from build123d import *

# Parameters (mm, degrees)
SKETCH_1_W          = 60
SKETCH_1_H          = 110
EXTRUDE_1_DEPTH     = 10
SKETCH_2_W          = 10
SKETCH_2_H          = 110
EXTRUDE_2_DEPTH     = 85
CUT_EXTRUDE_1_DEPTH = 85
SKETCH_4_R          = 26
EXTRUDE_3_DEPTH     = 21
CUT_EXTRUDE_2_DEPTH = 42
SKETCH_6_R          = 32
EXTRUDE_4_DEPTH     = 10
SKETCH_7_R          = 17.5
CUT_EXTRUDE_3_DEPTH = 81


with BuildPart() as part:
    # 스케치1 → 보스-돌출1 (new body)
    with BuildSketch(Plane(origin=(0, 0, 0), x_dir=(1, 0, 0), z_dir=(0, 1, 0))):
        Rectangle(SKETCH_1_W, SKETCH_1_H)
    extrude(amount=EXTRUDE_1_DEPTH)

    # 스케치2 → 보스-돌출2 (add)
    with BuildSketch(Plane(origin=(0, 10, 0), x_dir=(1, 0, 0), z_dir=(0, 1, 0))):
        Rectangle(SKETCH_2_W, SKETCH_2_H)
    extrude(amount=EXTRUDE_2_DEPTH)

    # 스케치3 → 컷-돌출1 (cut)
    with BuildSketch(Plane(origin=(5, 0, 0), x_dir=(0, 0, -1), z_dir=(1, 0, 0))):
        Polygon((-55, 10), (-1.927245104, 101.924707978), (-74.670847317, 101.924707978), (-74.670847317, 10), align=None)
    cut_extrude_1 = extrude(amount=-CUT_EXTRUDE_1_DEPTH, mode=Mode.SUBTRACT)

    # 대칭 복사1: 컷-돌출1 across plane
    add(cut_extrude_1.mirror(Plane.XY), mode=Mode.SUBTRACT)

    # 스케치4 → 보스-돌출3 (add, symmetric)
    with BuildSketch(Plane(origin=(0, 0, 0), x_dir=(0, 0, -1), z_dir=(1, 0, 0))):
        with Locations((0, 66)):
            Circle(SKETCH_4_R)
    extrude(amount=EXTRUDE_3_DEPTH, both=True)

    # 스케치5 → 컷-돌출2 (cut)
    with BuildSketch(Plane(origin=(21, 0, 0), x_dir=(0, 0, -1), z_dir=(1, 0, 0))):
        with BuildLine():
            Line((-16.854508663, 85.797109328), (-12.442891348, 105.747158049))
            Line((-12.442891348, 105.747158049), (16.049526521, 102.320854634))
            Line((16.049526521, 102.320854634), (20.027337967, 82.58028148))
            ThreePointArc((20.027337967, 82.58028148), (2.259138508, 91.901665838), (-16.854508663, 85.797109328))
        make_face()
    extrude(amount=-CUT_EXTRUDE_2_DEPTH, mode=Mode.SUBTRACT)

    # 스케치6 → 보스-돌출4 (add)
    with BuildSketch(Plane(origin=(21, 0, 0), x_dir=(0, 0, -1), z_dir=(1, 0, 0))):
        with Locations((0, 66)):
            Circle(SKETCH_6_R)
    extrude_4 = extrude(amount=EXTRUDE_4_DEPTH)

    # 대칭 복사2: 보스-돌출4 across plane
    add(extrude_4.mirror(Plane(origin=(0, 0, 0), x_dir=(0, 0, 1), z_dir=(1, 0, 0))))

    # 스케치7 → 컷-돌출3 (cut)
    with BuildSketch(Plane(origin=(31, 0, 0), x_dir=(0, 0, -1), z_dir=(1, 0, 0))):
        with Locations((0, 64.96726993)):
            Circle(SKETCH_7_R)
    extrude(amount=-CUT_EXTRUDE_3_DEPTH, mode=Mode.SUBTRACT)


solid = part.part
For this review, take the finished solid that the model builds, in its own axes (mm). A direction names the side the tool comes from. Round coordinates to 2 decimals unless told otherwise and drop trailing zeros. Loops run counter-clockwise (first coordinate to the right, second up) from the corner with the lowest first, then second, coordinate; pieces in that order, holes last. Notation, with made-up numbers: (6, 84) - (64, 84) arc R22 ccw to (64, 92) - close; hole circle Ø9 at (-23.75, 37.25). An arc over 180 degrees is marked (long way). Answer as CSV lines item,"result".
(1) Consider section C-C on y = 72.5. Give the boundary of the cut face in (x, z), then the cut area to 3 significant figures.
Checked values:
outline,"(-31, -31.33) - (-21, -31.33) - (-21, -25.17) - (21, -25.17) - (21, -31.33) - (31, -31.33) - (31, -15.8) - (-31, -15.8) - close; (-31, 15.8) - (31, 15.8) - (31, 31.33) - (21, 31.33) - (21, 25.17) - (-21, 25.17) - (-21, 31.33) - (-31, 31.33) - close"
area,"1,410 mm2"
(2) Consider section B-B on x = 8. Give the boundary of the cut face in (y, z), then the cut area to 3 significant figures.
Checked values:
outline,"(0, -55) - (10, -55) - (10, 55) - (0, 55) - close; circle Ø52 at (66, 0); hole circle Ø35 at (64.97, 0)"
area,"2,260 mm2"
(3) Mouldability with a two-part tool opening along X and no side actions: class faces 1 (the face through (31, 52, -14)), 2 (the face through (0, 5, -55)), 3 (the face through (-21, 92.2, 0.1)) as +X half, -X half, draft (parallel to the pull), parting line (faces both ways), or undercut.
Checked values:
face 1,"+X half"
face 2,"draft"
face 3,"undercut"
(4) Consider section D-D on z = -27.5. Give the boundary of the cut face in (x, y), then the cut area to 3 significant figures.
Checked values:
outline,"(-31, 49.64) - (-21, 49.64) - (-21, 82.36) - (-31, 82.36) - close; (-30, 0) - (30, 0) - (30, 10) - (5, 10) - (5, 57.63) - (-5, 57.63) - (-5, 10) - (-30, 10) - close; (21, 49.64) - (31, 49.64) - (31, 82.36) - (21, 82.36) - close"
area,"1,730 mm2"
(5) Wall thickness on line 1 (Y direction, x = 14.5, z = 0); line 2 (X direction, y = 47, z = 20); line 3 (Y direction, x = 6.5, z = 8): over which ranges is each line inside the solid? List them lowest first.
Checked values:
line 1,"y = 0 to 10, 40 to 47.47, 82.47 to 92"
line 2,"x = -31 to -21, -5 to 5, 21 to 31"
line 3,"y = 0 to 10, 41.26 to 49.4, 80.53 to 90.74"
(6) Tool access review of faces 4 (the face through (-30, 5, 1)), 5 (the face through (21, 92.2, 0.1)), 6 (the face through (-18, 10, -1)): name each direction out of +Z, -Z, +X, -X, +Y, -Y from which nothing blocks a thin tool from reaching the whole face with its end or side.
Checked values:
face 4,"+Z, -Z, -X, -Y"
face 5,"none"
face 6,"+Z, -Z, -X"
(7) Consider section A-A on z = 0. Give the boundary of the cut face in (x, y).
Checked values:
outline,"(-31, 34) - (-21, 34) - (-21, 40) - (-5, 40) - (-5, 10) - (-30, 10) - (-30, 0) - (30, 0) - (30, 10) - (5, 10) - (5, 40) - (21, 40) - (21, 34) - (31, 34) - (31, 47.47) - (-31, 47.47) - close; (-31, 82.47) - (31, 82.47) - (31, 98) - (21, 98) - (21, 92) - (-21, 92) - (-21, 98) - (-31, 98) - close"
(8) Insertion check: P1, Ø1.5, axis at x = -21.5, y = 71.5, coming from the +Z side; P2, Ø1, axis at x = -2.5, y = 80, coming from the -Z side; P3, Ø12.5, axis at x = -15.5, z = 11, coming from the +Y side. Each pin has a flat end and moves straight along its axis. Give the tip position at first contact, or say it passes through.
Checked values:
P1,"stops at z = 31.65"
P2,"stops at z = -22.22"
P3,"stops at y = 96.98"
